Could you check a few things on this model? Use its own coordinates, in mm. Face numbers are marked on the shaded views. Coordinates: 2 decimals unless noted, no trailing zeros. Loops run counter-clockwise (first coordinate to the right, second up) from the corner with the lowest first, then second, coordinate; pieces in that order, holes last. Notation, with made-up numbers: (58.25, 79.5) - (109.25, 79.5) arc R20 ccw to (109.25, 111.5) - close; hole circle Ø8 at (-16.75, 6). An arc over 180 degrees is marked (long way). One line per question, with ' | ' between items. Start each with the question number.
1. I want a section at D-D, the plane x = 16. Write out the boundary of the cut face in (y, z).
2. We'd pull the mould along X, two halves only. Please class the marked faces 1 and 2: pulls with the +X half, pulls with the -X half, needs draft (parallel to the pull), parting line crosses it, or undercut.
3. I want a section at B-B, the plane z = -0.5. Write out the boundary of the cut face in (x, y), then the cut area to 3 significant figures.
4. I want a section at A-A, the plane z = -4.5. Write out the boundary of the cut face in (x, y) (3 decimals), then the cut area to 3 significant figures.
5. I'm going to push flat-ended pins straight in: P1, Ø4, axis at x = 1, y = 3, coming from the -Z side (3 decimals); P2, Ø1, axis at y = 1, z = 1.5, coming from the -X side. Where does each tip first touch, or does it pass through?
6. Please list where these lines run through material, in increasing order: L1, parallel to X at y = 4, z = 0 (3 decimals); L2, parallel to X at y = 3.75, z = -1.5; L3, parallel to Z at x = -17, y = 7.5 (3 decimals). Write a range as [from, to].
7. I want a section at C-C, the plane x = -17. Write out the boundary of the cut face in (y, z) (3 decimals), then the cut area to 3 significant figures.
from build123d import *

# Parameters (mm, degrees)
BOSS_EXTRUDE1_DEPTH = 10


with BuildPart() as part:
    # Sketch1 → Boss-Extrude1 (new body)
    with BuildSketch(Plane(origin=(0, 0, 0), x_dir=(1, 0, 0), z_dir=(0, 1, 0))):
        with BuildLine():
            ThreePointArc((-11.409830056, -0.625), (-11.472615091, -1.043379639), (-11.566667227, -1.455857129))
            ThreePointArc((-11.566667227, -1.455857129), (-11.876370495, -2.321431821), (-12.322928267, -3.125))
            Line((-12.322928267, -3.125), (0, -3.125))
            Line((0, -3.125), (0, -0.625))
            Line((0, -0.625), (-11.409830056, -0.625))
        make_face()
        with BuildLine():
            Line((-11.566667227, -1.455857129), (-13.981481793, -0.808809516))
            ThreePointArc((-13.981481793, -0.808809516), (-14.004369338, -0.88984377), (-14.029431878, -0.970231948))
            add(Edge.make_bspline(
                [(-12.322928267, -3.125), (-14.629677343, -3.130705569), (-14.029431878, -0.970231948)],
                knots=[0, 0, 0, 0.964614565, 0.964614565, 0.964614565], degree=2))
            ThreePointArc((-12.322928267, -3.125), (-11.876370495, -2.321431821), (-11.566667227, -1.455857129))
        make_face()
        with BuildLine():
            Line((-22.433332773, -1.455857129), (-20.018518207, -0.808809516))
            ThreePointArc((-20.018518207, -0.808809516), (-17.407894351, 3.098265192), (-13.875, 0))
            ThreePointArc((-13.875, 0), (-13.901734808, -0.407894351), (-13.981481793, -0.808809516))
            Line((-13.981481793, -0.808809516), (-11.566667227, -1.455857129))
            ThreePointArc((-11.566667227, -1.455857129), (-11.472615091, -1.043379639), (-11.409830056, -0.625))
            ThreePointArc((-11.409830056, -0.625), (-11.383714264, -0.312984877), (-11.375, 0))
            ThreePointArc((-11.375, 0), (-17.734209831, 5.576877345), (-22.433332773, -1.455857129))
        make_face()
    boss_extrude1 = extrude(amount=BOSS_EXTRUDE1_DEPTH)

    # Mirror1: Boss-Extrude1 across plane
    add(boss_extrude1.mirror(Plane(origin=(0, 0, 0), x_dir=(0, 0, 1), z_dir=(1, 0, 0))))


solid = part.part
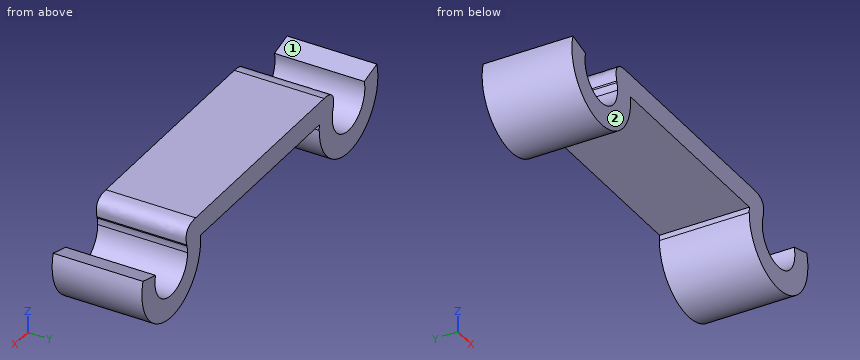
Results are:
1) outline: (0, -5.54) - (10, -5.54) - (10, -2.96) - (0, -2.96) - close
2) face 1: undercut | face 2: needs draft
3) outline: (-22.6, 0) - (-20.08, 0) - (-20.08, 10) - (-22.6, 10) - close; (-13.92, 0) - (-11.4, 0) - (-11.4, 10) - (-13.92, 10) - close; (11.4, 0) - (13.92, 0) - (13.92, 10) - (11.4, 10) - close; (20.08, 0) - (22.6, 0) - (22.6, 10) - (20.08, 10) - close | area: 101 mm2
4) outline: (-20.375, 0) - (-13.625, 0) - (-13.625, 10) - (-20.375, 10) - close; (13.625, 0) - (20.375, 0) - (20.375, 10) - (13.625, 10) - close | area: 135 mm2
5) P1: stops at z = 0.625 | P2: stops at x = -22.54
6) L1: x = [-22.625, -20.125], [-13.875, -11.375], [11.375, 13.875], [20.125, 22.625] | L2: x = [-22.42, -19.74], [-14.26, -11.58], [11.58, 14.26], [19.74, 22.42] | L3: z = [-5.625, -3.125]
7) outline: (0, -5.625) - (10, -5.625) - (10, -3.125) - (0, -3.125) - close | area: 25.0 mm2
